Autodesk Fusion 360 part; units mm, degrees
sketch "スケッチ1" plane through (0, 0, 0) normal (0, 0, 1) x (1, 0, 0)
  line L0 (0, 50) -> (0, -50)
  line L1 (100, -50) -> (100, 50)
  line L2 (8, -50) -> (8, -11)
  line L3 (0, -50) -> (8, -50)
  line L4 (92, -11) -> (92, -50)
  line L5 (92, -50) -> (100, -50)
  line L6 (84, 3) -> (16, 3)
  line L7 (16, -3) -> (84, -3)
  line L8 (8, 11) -> (8, 50)
  line L9 (8, 50) -> (0, 50)
  line L10 (92, 50) -> (92, 11)
  line L11 (100, 50) -> (92, 50)
  arc A0 (16, -3) -> (8, -11) centre (16, -11) ccw
  arc A1 (8, 11) -> (16, 3) centre (16, 11) ccw
  arc A2 (84, 3) -> (92, 11) centre (84, 11) ccw
  arc A3 (92, -11) -> (84, -3) centre (84, -11) ccw
extrude "押し出し1" add sketch "スケッチ1" along normal blind 100
CAD build for the part. Positions are in the model's coordinates, mm. A direction names the side the tool comes from. Coordinates: 2 decimals unless noted, no trailing zeros. Order: outer loops, then holes, each group sorted by start corner. A loop starts at its lowest first (then second) coordinate and runs counter-clockwise, first axis right, second up. Notation, with made-up numbers: (-3, -9) - (10, -9) arc R30 cw to (10, 30) - close; hole circle Ø8 at (-34, -2). An arc over 180 degrees is marked (long way). Answer in a Markdown table with one row per item.
1. Slice it at C-C, the plane x = 27. List the corners of the cut face in (y, z), then the cut area to 3 significant figures.
Answer:
| item | result |
|---|---|
| outline | (-3, 0) - (3, 0) - (3, 100) - (-3, 100) - close |
| area | 600 mm² |
2. Pull direction X, two halves, no side cores. Call faces 4 (the face through (0, 1, 49)), 5 (the face through (100, -1, 49)), 6 (the face through (10.406, 5.281, 49.3)), 7 (the face through (50, 0, 100)): +X half, -X half, draft (parallel to the pull), parting line (faces both ways), or undercut.
Answer:
| item | result |
|---|---|
| face 4 | -X half |
| face 5 | +X half |
| face 6 | undercut |
| face 7 | draft |
3. Slice it at A-A, the plane y = -15. List the corners of the cut face in (x, z).
Answer:
| item | result |
|---|---|
| outline | (0, 0) - (8, 0) - (8, 100) - (0, 100) - close; (92, 0) - (100, 0) - (100, 100) - (92, 100) - close |
4. Flat gauge pins, fed straight in: P1, Ø2, axis at x = 40, z = 37.5, coming from the -Y side; P2, Ø1.5, axis at x = 66, z = 20.5, coming from the +Y side; P3, Ø4, axis at x = 89, z = 61, coming from the +Y side; P4, Ø8, axis at x = 85, y = -14.5, coming from the -Z side. Where does each tip first touch, or does it go through?
Answer:
| item | result |
|---|---|
| P1 | y = -3 |
| P2 | y = 3 |
| P3 | y = 7.13 |
| P4 | through |
5. Drill centre lines: L1, parallel to X at y = 35.5, z = 65; L2, parallel to Y at x = 52.5, z = 26.5; L3, parallel to Y at x = 87.5, z = 52.5. Where is each one in solid material? Low to high. Write a range as from..to.
Answer:
| item | result |
|---|---|
| L1 | 0..8, 92..100 |
| L2 | -3..3 |
| L3 | -3.81..3.81 |
6. 3-axis set-ups, long thin cutter, end or side, ignore diameter. For faces 1 (the face through (92, -30, 49)), 2 (the face through (96, 50, 49)), 3 (the face through (50, 3, 49)): which of +Z, -Z, +X, -X, +Y, -Y reach the whole face in a straight line?
Answer:
| item | result |
|---|---|
| face 1 | +Z, -Z, -Y |
| face 2 | +Z, -Z, +X, -X, +Y |
| face 3 | +Z, -Z, +Y |
7. Slice it at B-B, the plane z = 91.5. List the corners of the cut face in (x, y).
Answer:
| item | result |
|---|---|
| outline | (0, -50) - (8, -50) - (8, -11) arc R8 cw to (16, -3) - (84, -3) arc R8 cw to (92, -11) - (92, -50) - (100, -50) - (100, 50) - (92, 50) - (92, 11) arc R8 cw to (84, 3) - (16, 3) arc R8 cw to (8, 11) - (8, 50) - (0, 50) - close |
